```python
from build123d import *

# Parameters (mm, degrees)
BOSS_EXTRUDE1_DEPTH   = 5
CUT_EXTRUDE1_DEPTH    = 86.941840799
BOSS_EXTRUDE6_DEPTH   = 5
BOSS_EXTRUDE6_2_DEPTH = 5
SKETCH4_W             = 28.34
SKETCH4_H             = 92
BOSS_EXTRUDE7_DEPTH   = 2
SKETCH5_R             = 2.6
CUT_EXTRUDE2_DEPTH    = 92.284319703
BOSS_EXTRUDE8_REACH   = 93.284
SKETCH6_R             = 4
SKETCH7_R             = 2.1
CUT_EXTRUDE4_DEPTH    = 92.284319703
BOSS_EXTRUDE9_START   = 5
SKETCH8_R             = 2.6
BOSS_EXTRUDE9_DEPTH   = 5


with BuildPart() as part:
    # Sketch1 → Boss-Extrude1 (new body)
    with BuildSketch(Plane(origin=(0, 0, 0), x_dir=(0, 0, -1), z_dir=(1, 0, 0))):
        Polygon((0, 0), (0, -81), (14.142135624, -66.857864376), (28.284271247, -81), (28.284271247, 0), (14.142135624, -14.142135624), align=None)
    extrude(amount=BOSS_EXTRUDE1_DEPTH)

    # Sketch2 → Cut-Extrude1 (cut, through all)
    with BuildSketch(Plane(origin=(5, 0, 0), x_dir=(0, 0, -1), z_dir=(1, 0, 0))):
        Polygon((4, -71.343145751), (12.142135624, -63.201010127), (12.142135624, -17.798989873), (4, -9.656854249), align=None)
        Polygon((16.142135624, -17.798989873), (16.142135624, -63.201010127), (24.284271247, -71.343145751), (24.284271247, -9.656854249), align=None)
    extrude(amount=-CUT_EXTRUDE1_DEPTH, mode=Mode.SUBTRACT)



with BuildPart() as body_2:
    # Sketch3 → Boss-Extrude6 (new body)
    with BuildSketch(Plane(origin=(5, 0, 0), x_dir=(0, 0, -1), z_dir=(1, 0, 0))):
        Polygon((-0.027864376, 3.619966825), (1.796051224, 1.796051224), (14.142135624, -10.550033175), (26.488220023, 1.796051224), (28.312135624, 3.619966825), (28.312135624, 5.5), (-0.027864376, 5.5), align=None)
    extrude(amount=-BOSS_EXTRUDE6_DEPTH)


with BuildPart() as body_3:
    # Sketch3 → Boss-Extrude6 2 (new body)
    with BuildSketch(Plane(origin=(5, 0, 0), x_dir=(0, 0, -1), z_dir=(1, 0, 0))):
        Polygon((14.142135624, -70.449966825), (1.796051224, -82.796051224), (-0.027864376, -84.619966825), (-0.027864376, -86.5), (28.312135624, -86.5), (28.312135624, -84.619966825), (26.488220023, -82.796051224), align=None)
    extrude(amount=-BOSS_EXTRUDE6_2_DEPTH)


with BuildPart() as part_1:
    add(part.part)

    add(body_2.part)  # Boss-Extrude7 merges body 2

    add(body_3.part)  # Boss-Extrude7 merges body 3
    # Sketch4 → Boss-Extrude7 (add)
    with BuildSketch(Plane.ZY):
        with Locations((-14.142135624, -40.5)):
            Rectangle(SKETCH4_W, SKETCH4_H)
    extrude(amount=BOSS_EXTRUDE7_DEPTH)

    # Sketch5 → Cut-Extrude2 (cut, through all)
    with BuildSketch(Plane(origin=(5, 0, 0), x_dir=(0, 0, -1), z_dir=(1, 0, 0))):
        with Locations((14.142135624, 0.3)):
            Circle(SKETCH5_R)
        with Locations(Location((14.142135624, -81.3, 0), (0, 0, 180))):
            Circle(SKETCH5_R)
    extrude(amount=-CUT_EXTRUDE2_DEPTH, mode=Mode.SUBTRACT)

    # Sketch6 → Boss-Extrude8 (add, up to next)
    with BuildSketch(Plane(origin=(5, 0, 0), x_dir=(0, 0, -1), z_dir=(1, 0, 0)), mode=Mode.PRIVATE) as boss_extrude8_sk1:
        with Locations((14.142135624, -55.5)):
            Circle(SKETCH6_R)
    boss_extrude8_tool1 = extrude(boss_extrude8_sk1.sketch, amount=-BOSS_EXTRUDE8_REACH, mode=Mode.PRIVATE) - part_1.part
    # Sketch6 → Boss-Extrude8 (add, up to next)
    with BuildSketch(Plane(origin=(5, 0, 0), x_dir=(0, 0, -1), z_dir=(1, 0, 0)), mode=Mode.PRIVATE) as boss_extrude8_sk2:
        with Locations((14.142135624, -25.5)):
            Circle(SKETCH6_R)
    boss_extrude8_tool2 = extrude(boss_extrude8_sk2.sketch, amount=-BOSS_EXTRUDE8_REACH, mode=Mode.PRIVATE) - part_1.part
    add(boss_extrude8_tool1.solids().sort_by_distance((5, -55.5, -14.142136))[0])
    add(boss_extrude8_tool1.solids().sort_by_distance((5, -55.5, -14.142136))[1])
    add(boss_extrude8_tool2.solids().sort_by_distance((5, -25.5, -14.142136))[0])
    add(boss_extrude8_tool2.solids().sort_by_distance((5, -25.5, -14.142136))[1])

    # Sketch7 → Cut-Extrude4 (cut, through all)
    with BuildSketch(Plane(origin=(5, 0, 0), x_dir=(0, 0, -1), z_dir=(1, 0, 0))):
        with Locations((14.142135624, -25.5)):
            Circle(SKETCH7_R)
        with Locations((14.142135624, -55.5)):
            Circle(SKETCH7_R)
    extrude(amount=-CUT_EXTRUDE4_DEPTH, mode=Mode.SUBTRACT)

    # Sketch8 → Boss-Extrude9 (add)
    # profile 1 of 2: a face of its own
    with BuildSketch(Plane(origin=(5, 0, 0), x_dir=(0, 0, -1), z_dir=(1, 0, 0)).offset(BOSS_EXTRUDE9_START)):
        Polygon((28.312135624, 5.5), (28.312135624, 3.619966825), (14.142135624, -10.550033175), (-0.027864376, 3.619966825), (-0.027864376, 5.5), align=None)
        with Locations((14.142135624, 0.3)):
            Circle(SKETCH8_R, mode=Mode.SUBTRACT)
    # profile 2 of 2: a face of its own
    with BuildSketch(Plane(origin=(5, 0, 0), x_dir=(0, 0, -1), z_dir=(1, 0, 0)).offset(BOSS_EXTRUDE9_START)):
        Polygon((28.312135624, -86.5), (28.312135624, -84.619966825), (14.142135624, -70.449966825), (-0.027864376, -84.619966825), (-0.027864376, -86.5), align=None)
        with Locations(Location((14.142135624, -81.3, 0), (0, 0, 180))):
            Circle(SKETCH8_R, mode=Mode.SUBTRACT)
    extrude(amount=-BOSS_EXTRUDE9_DEPTH)


solid = part_1.part
```
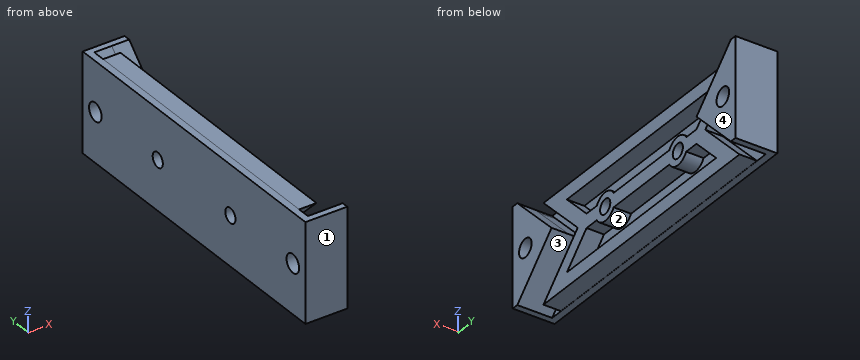
Can you work these out from the model? Positions are in its coordinate system, mm. Face numbers are marked on the shaded views. A direction names the side the tool comes from. Give positions to 0.01 mm unless a question says otherwise; leave off trailing zeros. Loops run counter-clockwise (first coordinate to the right, second up) from the corner with the lowest first, then second, coordinate; pieces in that order, holes last. Notation, with made-up numbers: M -25,-5.5 L 2,-5.5 A8 cw 2,7.5 Z; hole C 72,65.5 d3. An arc over 180 degrees is marked long. Answer in a Markdown table with one row per item.
1. Suppose I cut it at D-D on x = 3. Count the separate pieces of the cut face and the enclosed holes in it, plus the area to 3 significant figures.
Taken from the geometry:
| item | result |
|---|---|
| separate pieces | 3 |
| enclosed holes | 6 |
| area | 1,500 mm² |
2. For pin 1 Ø2.5 at (x, y) = (2, -20.5) entering from -Z; pin 2 Ø4 at (y, z) = (-66, -17.5) entering from +X; pin 3 Ø3.5 at (x, y) = (2.5, -62) entering from +Z, each with a flat end and sliding along its axis, tell me the tip position at first contact or that it passes through.
Taken from the geometry:
| item | result |
|---|---|
| pin 1 | stops at z = -28.28 |
| pin 2 | stops at x = 5 |
| pin 3 | stops at z = 0 |
3. Which directions (+Z, -Z, +X, -X, +Y, -Y) give clear straight access to the entire face, cutting with the end or side of a thin tool? Please do the marked faces 3 and 4.
Taken from the geometry:
| item | result |
|---|---|
| face 3 | +X |
| face 4 | +Z, -Z, +X, +Y, -Y |
4. If I drill on line 1 along Y through (x, z) = (-0.75, -14.25); line 2 along Y through (x, z) = (1.5, -6.25); line 3 along Y through (x, z) = (3, -20.75), over which ranges is the centre line in solid material (lowest first)?
Taken from the geometry:
| item | result |
|---|---|
| line 1 | y = -86.5 to -83.9, -78.7 to -57.6, -53.4 to -27.6, -23.4 to -2.3, 2.9 to 5.5 |
| line 2 | y = -86.5 to -78.34, -74.75 to -69.09, -11.91 to -6.25, -2.66 to 5.5 |
| line 3 | y = -86.5 to -77.06, -73.47 to -67.81, -13.19 to -7.53, -3.94 to 5.5 |
5. Thinking about a two-plate mould opening in Z: for the marked faces 1 and 2, which applies, released by +Z, released by -Z, zero draft, split by the parting line, or undercut?
Taken from the geometry:
| item | result |
|---|---|
| face 1 | zero draft |
| face 2 | undercut |
6. Suppose I cut it at A-A on x = 7. Write out the boundary of the cut face in (y, z).
Taken from the geometry:
| item | result |
|---|---|
| outline | M -86.5,-28.31 L -84.62,-28.31 L -70.45,-14.14 L -84.62,0.03 L -86.5,0.03 Z; M -10.55,-14.14 L 3.62,-28.31 L 5.5,-28.31 L 5.5,0.03 L 3.62,0.03 Z; hole C -81.3,-14.14 d5.2; hole C 0.3,-14.14 d5.2 |
